Verification items for the finished model (mm, model axes). A direction names the side the tool comes from. Give positions to 0.01 mm unless a question says otherwise; leave off trailing zeros. Write each loop counter-clockwise with the first axis right and the second up, starting at its lowest first coordinate (ties: lowest second). Pieces come first, ordered by that corner, then holes. Notation, with made-up numbers: (-31, 53.5) -> (-26, 53.5) arc R19 ccw to (-26, 59.5) -> close; hole circle Ø2 at (-18, -35.5). An arc over 180 degrees is marked (long way). Write item = value, one per line.
from build123d import *

# Parameters (mm, degrees)
SKETCH1_R           = 1.6
BOSS_EXTRUDE2_DEPTH = 3


with BuildPart() as part:
    # Sketch1 → Boss-Extrude2 (new body)
    with BuildSketch(Plane(origin=(0, 0, 0), x_dir=(1, 0, 0), z_dir=(0, 1, 0))):
        with BuildLine():
            Line((-70, 45), (70, 45))
            ThreePointArc((70, 45), (73.535533906, 43.535533906), (75, 40))
            Line((75, 40), (75, -40))
            ThreePointArc((75, -40), (73.535533906, -43.535533906), (70, -45))
            Line((70, -45), (-70, -45))
            ThreePointArc((-70, -45), (-73.535533906, -43.535533906), (-75, -40))
            Line((-75, -40), (-75, 40))
            ThreePointArc((-75, 40), (-73.535533906, 43.535533906), (-70, 45))
        make_face()
        with Locations(Location((16.25, 24.25, 0), (0, 0, 270))):
            Circle(SKETCH1_R, mode=Mode.SUBTRACT)
        with Locations(Location((58.75, 24.25, 0), (0, 0, 90))):
            Circle(SKETCH1_R, mode=Mode.SUBTRACT)
        with Locations(Location((58.75, -24.25, 0), (0, 0, 270))):
            Circle(SKETCH1_R, mode=Mode.SUBTRACT)
        with Locations(Location((16.25, -24.25, 0), (0, 0, 90))):
            Circle(SKETCH1_R, mode=Mode.SUBTRACT)
        with Locations(Location((-34.65, 27.81, 0), (0, 0, 270))):
            Circle(SKETCH1_R, mode=Mode.SUBTRACT)
        with Locations(Location((-15.35, 27.81, 0), (0, 0, 90))):
            Circle(SKETCH1_R, mode=Mode.SUBTRACT)
        with Locations(Location((-15.35, -27.81, 0), (0, 0, 270))):
            Circle(SKETCH1_R, mode=Mode.SUBTRACT)
        with Locations(Location((-34.65, -27.81, 0), (0, 0, 90))):
            Circle(SKETCH1_R, mode=Mode.SUBTRACT)
        with Locations(Location((-70, 40, 0), (0, 0, 270))):
            Circle(SKETCH1_R, mode=Mode.SUBTRACT)
        with Locations(Location((-70, -40, 0), (0, 0, 90))):
            Circle(SKETCH1_R, mode=Mode.SUBTRACT)
        with Locations(Location((70, 40, 0), (0, 0, 90))):
            Circle(SKETCH1_R, mode=Mode.SUBTRACT)
        with Locations(Location((70, -40, 0), (0, 0, 270))):
            Circle(SKETCH1_R, mode=Mode.SUBTRACT)
        with BuildLine():
            Line((33, 35), (42, 35))
            ThreePointArc((42, 35), (47.656854249, 32.656854249), (50, 27))
            Line((50, 27), (50, -27))
            ThreePointArc((50, -27), (47.656854249, -32.656854249), (42, -35))
            Line((42, -35), (33, -35))
            ThreePointArc((33, -35), (27.343145751, -32.656854249), (25, -27))
            Line((25, -27), (25, 27))
            ThreePointArc((25, 27), (27.343145751, 32.656854249), (33, 35))
        make_face(mode=Mode.SUBTRACT)
    extrude(amount=BOSS_EXTRUDE2_DEPTH)


solid = part.part
Item 1: Set-up check for faces 1 (the cylindrical face through (-73, 1, 44)), 2 (the cylindrical face through (27.406, 1.479, 32.719)): record each of +Z, -Z, +X, -X, +Y, -Y from which the full face is reachable in a straight line by a thin tool's end or side.
Response values:
face_1 = +Z, -X, +Y, -Y
face_2 = +Y, -Y
Item 2: Mould release check, pull along Z, two halves, no side actions. Record for faces 3 (the cylindrical face through (74, 1, 43)), 4 (the flat face through (1, 0, -1)), 5 (the cylindrical face through (-14.38, 1.48, -26.54)): +Z half, -Z half, draft (parallel to the pull), parting line (faces both ways), or undercut.
Response values:
face_3 = +Z half
face_4 = draft
face_5 = undercut
Item 3: Sectioned sample at A-A on x = -15.35. Record the cut outline in (y, z), then the cut area to 3 significant figures.
Response values:
outline = (0, -45) -> (3, -45) -> (3, -29.41) -> (0, -29.41) -> close; (0, -26.21) -> (3, -26.21) -> (3, 26.21) -> (0, 26.21) -> close; (0, 29.41) -> (3, 29.41) -> (3, 45) -> (0, 45) -> close
area = 251 mm^2
Item 4: Go/stop test with flat-tipped pins: P1, Ø4, axis at x = 16.25, z = 24.25, coming from the +Y side; P2, Ø1.9, axis at x = -34.65, z = 27.81, coming from the -Y side. Record where each tip stops, or that it passes through.
Response values:
P1 = 3
P2 = through
Item 5: Sectioned sample at D-D on y = 1.2. Give the number of separate pieces and of enclosed holes in the cut face, then the cut area to 3 significant figures.
Response values:
separate_pieces = 1
enclosed_holes = 13
area = 11,700 mm^2
Item 6: Sectioned sample at C-C on z = -10.5. Record the cut outline in (x, y), then the cut area to 3 significant figures.
Response values:
outline = (-75, 0) -> (25, 0) -> (25, 3) -> (-75, 3) -> close; (50, 0) -> (75, 0) -> (75, 3) -> (50, 3) -> close
area = 375 mm^2
Item 7: Sectioned sample at B-B on z = -24.25. Record the cut outline in (x, y), then the cut area to 3 significant figures.
Response values:
outline = (-75, 0) -> (14.65, 0) -> (14.65, 3) -> (-75, 3) -> close; (17.85, 0) -> (25, 0) -> (25, 3) -> (17.85, 3) -> close; (50, 0) -> (57.15, 0) -> (57.15, 3) -> (50, 3) -> close; (60.35, 0) -> (75, 0) -> (75, 3) -> (60.35, 3) -> close
area = 356 mm^2
Item 8: Material ranges on line 1 (Z direction, x = -70, y = 0.95); line 2 (X direction, y = 1.05, z = 24.5); line 3 (Z direction, x = 16.5, y = 2), recorded low to high.
Response values:
line_1 = -45 to -41.6, -38.4 to 38.4, 41.6 to 45
line_2 = -75 to 14.67, 17.83 to 25, 50 to 57.17, 60.33 to 75
line_3 = -45 to -25.83, -22.67 to 22.67, 25.83 to 45
